Geometry: see drawing. Coordinates: mm, zero at the bounding-box minimum. Round coordinates to 2 decimals unless told otherwise and drop trailing zeros. Order: outer loops, then holes, each group sorted by start corner. A loop starts at its lowest first (then second) coordinate and runs counter-clockwise, first axis right, second up. Notation, with made-up numbers: (82.25, 19.25) -> (124.25, 19.25) arc R32 cw to (124.25, 57.25) -> close; hole circle Ø9 at (62, 79.25). An arc over 180 degrees is marked (long way). Answer as CSV lines item,"result". Start each with the question number.
(1) Section query C-C (z = 9). Output: boundary loops of the cut face in (x, y).
(2) Pull-direction query (X, two-part tool) for the marked faces 1, 2, 3 and 4; classes: +X half, -X half, draft (parallel to the pull), parting line (faces both ways), or undercut.
(3) Contact query for a flat-ended pin moving along its axis: P1, Ø3, axis at x = 17, z = 3, coming from the +Y side. Output: stop coordinate, or through.
(4) Section query B-B (x = 30). Output: boundary loops of the cut face in (y, z).
(5) Line query: line 1 along X through (y, z) = (2.25, 8.5); line 2 along Z through (x, y) = (30, 6.25); line 3 along X through (y, z) = (6, 9). Output: solid intervals per line, ascending. Write a range as from..to.
(6) Section query A-A (y = 3). Output: boundary loops of the cut face in (x, z), plus the area to 3 significant figures.
(7) Section query D-D (z = 4.25). Output: boundary loops of the cut face in (x, y), plus the area to 3 significant figures.
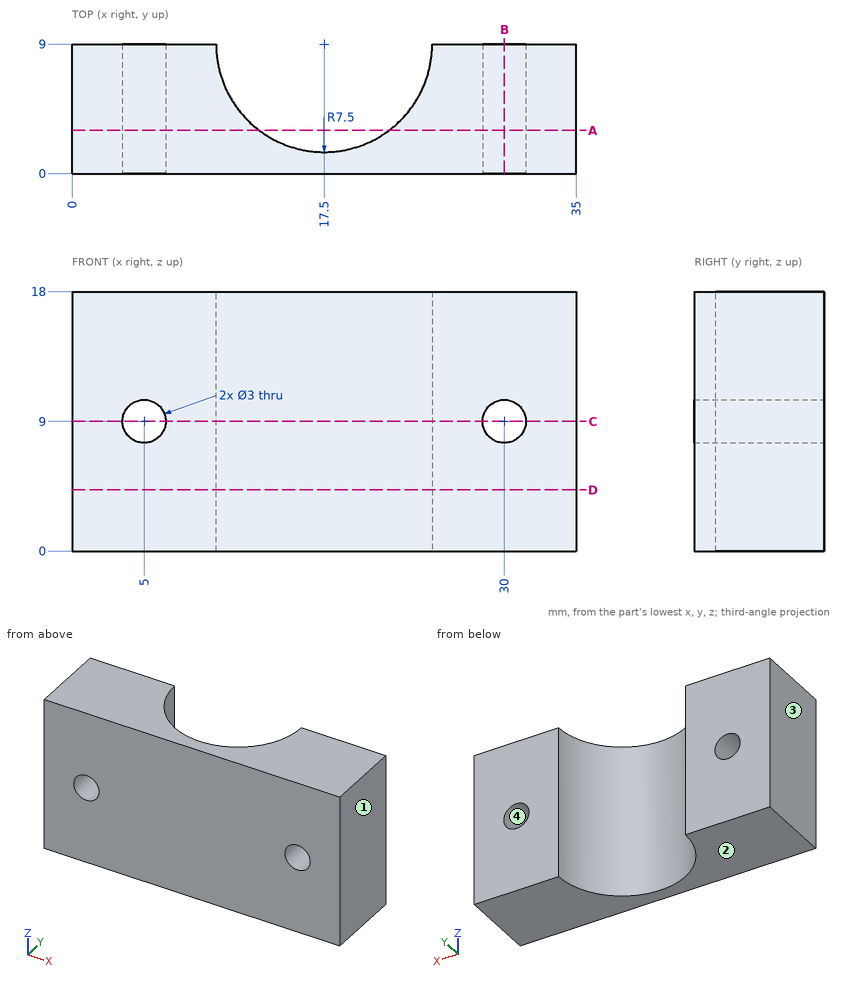
Answer block:
1,outline,"(0, 0) -> (3.5, 0) -> (3.5, 9) -> (0, 9) -> close; (6.5, 0) -> (28.5, 0) -> (28.5, 9) -> (25, 9) arc R7.5 cw to (10, 9) -> (6.5, 9) -> close; (31.5, 0) -> (35, 0) -> (35, 9) -> (31.5, 9) -> close"
2,face 1,"+X half"
2,face 2,"draft"
2,face 3,"-X half"
2,face 4,"undercut"
3,P1,"y = 1.77"
4,outline,"(0, 0) -> (9, 0) -> (9, 7.5) -> (0, 7.5) -> close; (0, 10.5) -> (9, 10.5) -> (9, 18) -> (0, 18) -> close"
5,line 1,"0..3.59, 6.41..14.23, 20.77..28.59, 31.41..35"
5,line 2,"0..7.5, 10.5..18"
5,line 3,"0..3.5, 6.5..10.63, 24.37..28.5, 31.5..35"
6,outline,"(0, 0) -> (13, 0) -> (13, 18) -> (0, 18) -> close; (22, 0) -> (35, 0) -> (35, 18) -> (22, 18) -> close; hole circle Ø3 at (5, 9); hole circle Ø3 at (30, 9)"
6,area,"454 mm2"
7,outline,"(0, 0) -> (35, 0) -> (35, 9) -> (25, 9) arc R7.5 cw to (10, 9) -> (0, 9) -> close"
7,area,"227 mm2"
